```python
from build123d import *

# Parameters (mm, degrees)
BOSS_EXTRUDE1_DEPTH     = 120.65
SKETCH5_R               = 0.55245
CUT_EXTRUDE1_DEPTH      = 121.65
CUT_EXTRUDE1_DEPTH_BACK = 121.65


with BuildPart() as part:
    # Sketch4 → Boss-Extrude1 (new body, symmetric)
    with BuildSketch(Plane.XY):
        with BuildLine():
            Line((4.190365, -12.7), (10.11729625, -12.7))
            ThreePointArc((10.11729625, -12.7), (11.943543585, -11.943543585), (12.7, -10.11729625))
            Line((12.7, -10.11729625), (12.7, -4.190365))
            ThreePointArc((12.7, -4.190365), (12.42492494, -3.52627506), (11.760835, -3.2512))
            Line((11.760835, -3.2512), (11.429365, -3.2512))
            ThreePointArc((11.429365, -3.2512), (10.76527506, -3.52627506), (10.4902, -4.190365))
            Line((10.4902, -4.190365), (10.4902, -6.348478019))
            ThreePointArc((10.4902, -6.348478019), (9.830707141, -7.335478831), (8.666460301, -7.103895736))
            Line((8.666460301, -7.103895736), (5.299899128, -3.737334563))
            ThreePointArc((5.299899128, -3.737334563), (4.817571085, -3.015479634), (4.6482, -2.16399369))
            Line((4.6482, -2.16399369), (4.6482, 0))
            Line((4.6482, 0), (2.6035, 0))
            ThreePointArc((2.6035, 0), (1.840952505, -1.840952505), (0, -2.6035))
            Line((0, -2.6035), (0, -4.6482))
            Line((0, -4.6482), (2.16399369, -4.6482))
            ThreePointArc((2.16399369, -4.6482), (3.015479634, -4.817571085), (3.737334563, -5.299899128))
            Line((3.737334563, -5.299899128), (7.103895736, -8.666460301))
            ThreePointArc((7.103895736, -8.666460301), (7.335478831, -9.830707141), (6.348478019, -10.4902))
            Line((6.348478019, -10.4902), (4.190365, -10.4902))
            ThreePointArc((4.190365, -10.4902), (3.52627506, -10.76527506), (3.2512, -11.429365))
            Line((3.2512, -11.429365), (3.2512, -11.760835))
            ThreePointArc((3.2512, -11.760835), (3.52627506, -12.42492494), (4.190365, -12.7))
        make_face()
    extrude(amount=BOSS_EXTRUDE1_DEPTH, both=True)

    # Sketch5 → Cut-Extrude1 (cut, two sides)
    with BuildSketch(Plane.XY) as cut_extrude1_sk:
        with Locations((10.356153152, -12.7)):
            Circle(SKETCH5_R)
        with Locations((5.796028019, -12.7)):
            Circle(SKETCH5_R)
        with Locations((12.7, -10.356153152)):
            Circle(SKETCH5_R)
        with Locations((12.7, -5.796028019)):
            Circle(SKETCH5_R)
    extrude(amount=CUT_EXTRUDE1_DEPTH, mode=Mode.SUBTRACT)
    extrude(cut_extrude1_sk.sketch, amount=-CUT_EXTRUDE1_DEPTH_BACK, mode=Mode.SUBTRACT)

    # Mirror1: part across plane


with BuildPart() as part_1:
    add(part.part)
    add(part.part.mirror(Plane(origin=(0, 0, 0), x_dir=(0, 0, 1), z_dir=(1, 0, 0))))

    # Mirror2: part across plane


with BuildPart() as part_2:
    add(part_1.part)
    add(part_1.part.mirror(Plane.ZX))


solid = part_2.part
```
Part model, mm, in its own coordinate system. A direction names the side the tool comes from. Coordinates: 2 decimals unless noted, no trailing zeros. Write item = value, one per line. Start each with the question number.
Item 1: Mould opens along Y. For faces 1 (the flat face through (4.648, 0, 2)), 2 (the flat face through (0, -4.648, 2)), 3 (the flat face through (0, -3, 120.65)) say: released by +Y, released by -Y, zero draft, split by the parting line, or undercut.
Item 2: 3-axis set-ups, long thin cutter, end or side, ignore diameter. For faces 4 (the flat face through (0, 4.648, 2)), 5 (the flat face through (-4.648, 0, 2)), 6 (the flat face through (0, -3, -120.65)): which of +Z, -Z, +X, -X, +Y, -Y reach the whole face in a straight line?
Item 3: Wall check: L1, parallel to X at y = 4.5, z = -53.5; L2, parallel to X at y = -0.5, z = 3; L3, parallel to Y at x = 3.75, z = 102.5. Give the ranges that are in metal, low to high. Write a range as from..to.
Item 4: Flat gauge pins, fed straight in: pin 1 Ø3.5 at (y, z) = (0.5, -57.5) entering from +X; pin 2 Ø4 at (x, z) = (-5.5, 11.5) entering from -Y; pin 3 Ø4 at (y, z) = (-1, -13) entering from -X; pin 4 Ø6 at (y, z) = (-0.5, 78.5) entering from +X. Where does each tip first touch, or does it go through?
The answers:
q1.face_1 = undercut
q1.face_2 = released by -Y
q1.face_3 = zero draft
q2.face_4 = +Z, -Z, +Y
q2.face_5 = +Z, -Z, -X
q2.face_6 = -Z, +X, -X, +Y, -Y
q3.L1 = -12.7..-10.49, -6.06..6.06, 10.49..12.7
q3.L2 = -4.65..-2.56, 2.56..4.65
q3.L3 = -12.59..-10.6, -5.31..5.31, 10.6..12.59
q4.pin_1 = 4.65
q4.pin_2 = -12.7
q4.pin_3 = -4.81
q4.pin_4 = 12.4
